Can you work these out from the model? Positions are in its coordinate system, mm. Give positions to 0.01 mm unless a question says otherwise; leave off trailing zeros. Order: outer loops, then holes, each group sorted by start corner. A loop starts at its lowest first (then second) coordinate and runs counter-clockwise, first axis right, second up.
Item 1: I want a section at B-B, the plane y = 13.5. Write out the boundary of the cut face in (x, z), then the cut area to 3 significant figures.
Item 2: I want a section at A-A, the plane y = -12.5. Write out the boundary of the cut face in (x, z).
Item 3: I'm going to push flat-ended pins straight in: pin 1 Ø12 at (x, y) = (3.5, -15.5) entering from -Z; pin 2 Ø2 at (y, z) = (-18.5, 1) entering from +X; pin 3 Ø12 at (x, y) = (7, 11.5) entering from +Z. Where does each tip first touch, or does it pass through?
Item 4: I want a section at C-C, the plane y = 20. Write out the boundary of the cut face in (x, z).
```python
from build123d import *

# Parameters (mm, degrees)
CYLINDER001_R       = 18
CYLINDER001_DEPTH   = 10
CYLINDER_R          = 25
CYLINDER_DEPTH      = 0.1
CUT_PLACEMENT_ANGLE = 5


with BuildPart() as cylinder001:
    # Cylinder001 → Cylinder001 (new body)
    with BuildSketch(Plane.XY):
        Circle(CYLINDER001_R)
    extrude(amount=CYLINDER001_DEPTH)


with BuildPart() as cut:
    # Cylinder → Cylinder (new body)
    with BuildSketch(Plane.XY):
        Circle(CYLINDER_R)
    extrude(amount=CYLINDER_DEPTH)

    # Cut: cut Cylinder001
    add(cylinder001.part, mode=Mode.SUBTRACT)


with BuildPart() as cut_1:
    # Cut placement: moved
    add(cut.part.rotate(Axis((0, 0, 0), (0, -1, 0)), CUT_PLACEMENT_ANGLE))


solid = cut_1.part
```
Results list:
1. outline: (-20.97, -1.73) - (-20.96, -1.83) - (-11.86, -1.04) - (-11.87, -0.94) - close; (11.85, 1.14) - (11.86, 1.04) - (20.96, 1.83) - (20.95, 1.93) - close
1. area: 1.83 mm2
2. outline: (-21.58, -1.79) - (-21.57, -1.89) - (-12.9, -1.13) - (-12.91, -1.03) - close; (12.89, 1.23) - (12.9, 1.13) - (21.57, 1.89) - (21.56, 1.99) - close
3. pin 1: stops at z = -0.18
3. pin 2: stops at x = 17.63
3. pin 3: stops at z = 1.23
4. outline: (-14.95, -1.21) - (-14.94, -1.31) - (14.94, 1.31) - (14.93, 1.41) - close
